```python
from build123d import *

# Parameters (mm, degrees)
BOSS_EXTRUDE1_DEPTH = 30
SKETCH2_R           = 2.25
CUT_EXTRUDE1_DEPTH  = 40.05124838
SKETCH3_R           = 2.25
CUT_EXTRUDE2_DEPTH  = 40.05124838


with BuildPart() as part:
    # Sketch1 → Boss-Extrude1 (new body)
    with BuildSketch(Plane(origin=(0, 0, 0), x_dir=(0, 0, -1), z_dir=(1, 0, 0))):
        Polygon((0, 0), (0, 20), (-5, 20), (-5, 5), (-20, 5), (-20, 0), align=None)
    extrude(amount=BOSS_EXTRUDE1_DEPTH)

    # Sketch2 → Cut-Extrude1 (cut, through all)
    with BuildSketch(Plane.XY.offset(5)):
        with Locations((7.5, 12.5)):
            Circle(SKETCH2_R)
        with Locations((22.5, 12.5)):
            Circle(SKETCH2_R)
    extrude(amount=-CUT_EXTRUDE1_DEPTH, mode=Mode.SUBTRACT)

    # Sketch3 → Cut-Extrude2 (cut, through all)
    with BuildSketch(Plane(origin=(0, 5, 0), x_dir=(1, 0, 0), z_dir=(0, 1, 0))):
        with Locations(Location((7.5, -12.5, 0), (0, 0, 270))):
            Circle(SKETCH3_R)
        with Locations(Location((22.5, -12.5, 0), (0, 0, 270))):
            Circle(SKETCH3_R)
    extrude(amount=-CUT_EXTRUDE2_DEPTH, mode=Mode.SUBTRACT)


solid = part.part
```
Here's how the part is built. I have some questions about the finished solid (model axes, mm). A direction names the side the tool comes from. Coordinates: 2 decimals unless noted, no trailing zeros. Loops run counter-clockwise (first coordinate to the right, second up) from the corner with the lowest first, then second, coordinate; pieces in that order, holes last. Notation, with made-up numbers: M 41,-23 L 59,-23 A19 ccw 59,0 Z; hole C -39,-7 d10. An arc over 180 degrees is marked long. One line per item, written item: value.
1. Imagine slicing it at B-B (y = 12.5). List the corners of the cut face in (x, z) for me.
Geometry says:
outline: M 0,0 L 5.25,0 L 5.25,5 L 0,5 Z; M 9.75,0 L 20.25,0 L 20.25,5 L 9.75,5 Z; M 24.75,0 L 30,0 L 30,5 L 24.75,5 Z
2. Imagine slicing it at A-A (x = 7.5). List the corners of the cut face in (y, z) for me.
Geometry says:
outline: M 0,0 L 10.25,0 L 10.25,5 L 5,5 L 5,10.25 L 0,10.25 Z; M 0,14.75 L 5,14.75 L 5,20 L 0,20 Z; M 14.75,0 L 20,0 L 20,5 L 14.75,5 Z
3. Imagine slicing it at C-C (x = 27.25). List the corners of the cut face in (y, z) for me, and give its area (3 significant figures).
Geometry says:
outline: M 0,0 L 20,0 L 20,5 L 5,5 L 5,20 L 0,20 Z
area: 175 mm2
4. Thinking about a two-plate mould opening in X: for faces 1 (the flat face through (15, 5, 12)), 2 (the flat face through (0, 6, 3)), 3 (the cylindrical face through (7.21, 14.73, 2.54)), which applies, +X half, -X half, draft (parallel to the pull), parting line (faces both ways), or undercut?
Geometry says:
face 1: draft
face 2: -X half
face 3: undercut
5. Imagine slicing it at D-D (z = 18.25). List the corners of the cut face in (x, y) for me, and give its area (3 significant figures).
Geometry says:
outline: M 0,0 L 30,0 L 30,5 L 0,5 Z
area: 150 mm2
6. Will these pins go through, and if not, where does the flat tip stop? pin 1 Ø7 at (x, z) = (7.5, 12.5) entering from +Y; pin 2 Ø7 at (x, y) = (22.5, 12.5) entering from +Z.
Geometry says:
pin 1: stops at y = 5
pin 2: stops at z = 5
7. Please list where these lines run through material, in increasing order: probe 1 along X at (y, z) = (1.1, 12.5); probe 2 along Y at (x, z) = (22.5, 3.6); probe 3 along Z at (x, y) = (3.25, 13).
Geometry says:
probe 1: x = 0 to 5.25, 9.75 to 20.25, 24.75 to 30
probe 2: y = 0 to 10.25, 14.75 to 20
probe 3: z = 0 to 5
8. On a 3-axis mill with a long thin cutter (end or side, diameter ignored), from which of +Z, -Z, +X, -X, +Y, -Y can I reach the whole of each face in a straight line? I mean faces 4 (the flat face through (15, 20, 2)), 5 (the flat face through (15, 13, 5)). Say none if no direction works.
Geometry says:
face 4: +Z, -Z, +X, -X, +Y
face 5: +Z, +X, -X, +Y
